Verification items for this drawing (mm, ordinates from the low corner). Round coordinates to 2 decimals unless told otherwise and drop trailing zeros. Order: outer loops, then holes, each group sorted by start corner. A loop starts at its lowest first (then second) coordinate and runs counter-clockwise, first axis right, second up. Notation, with made-up numbers: (-21.75, 28.25) - (5.25, 28.25) arc R10 cw to (5.25, 37.25) - close; hole circle Ø11 at (-8.5, 0). An arc over 180 degrees is marked (long way). Return JSON: item names as keys, results as strings. Group by question number.
Q1. Sectioned sample at C-C, the plane x = 8. Record the cut outline in (y, z), then the cut area to 3 significant figures.
Q2. Material ranges on line 1 along Y through (x, z) = (65, 1); line 2 along Y through (x, z) = (23.5, 0.75) (1 decimal); line 3 along X through (y, z) = (103, 1.4) (1 decimal), recorded low to high.
Q3. Sectioned sample at A-A, the plane y = 65. Record the cut outline in (x, z).
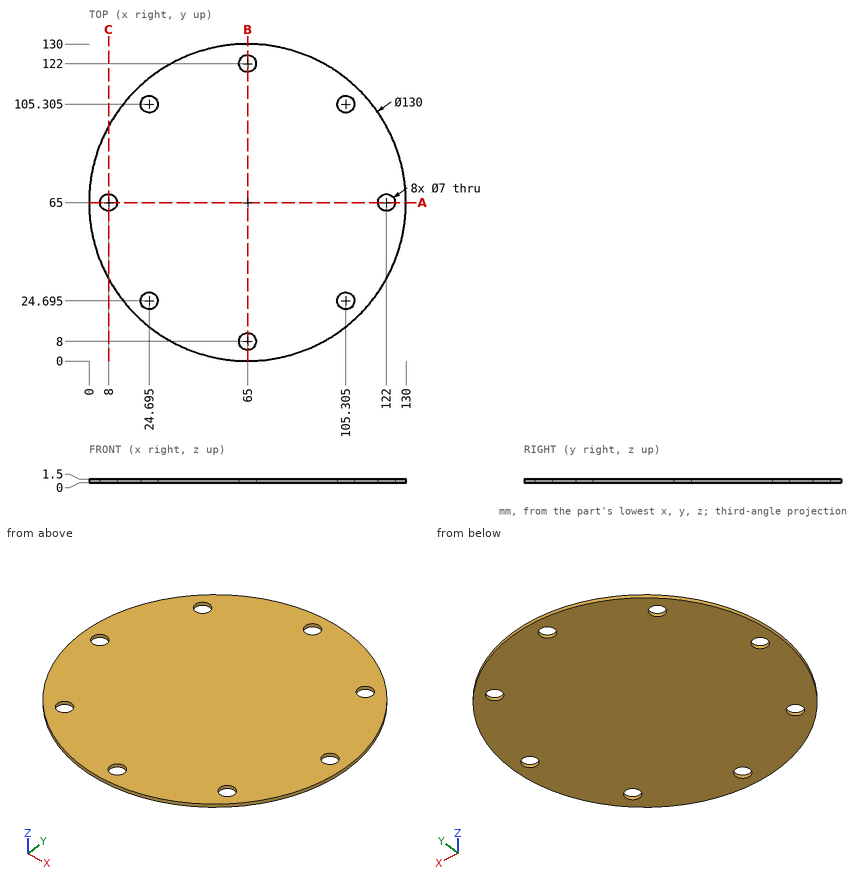
Reply:
{
 "1": {"outline": "(33.76, 0) - (61.5, 0) - (61.5, 1.5) - (33.76, 1.5) - close; (68.5, 0) - (96.24, 0) - (96.24, 1.5) - (68.5, 1.5) - close", "area": "83.2 mm^2"},
 "2": {"line 1": "0 to 4.5, 11.5 to 118.5, 125.5 to 130", "line 2": "15 to 21.4, 28 to 102, 108.6 to 115", "line 3": "12.3 to 22.1, 27.3 to 102.7, 107.9 to 117.7"},
 "3": {"outline": "(0, 0) - (4.5, 0) - (4.5, 1.5) - (0, 1.5) - close; (11.5, 0) - (118.5, 0) - (118.5, 1.5) - (11.5, 1.5) - close; (125.5, 0) - (130, 0) - (130, 1.5) - (125.5, 1.5) - close"}
}
